The model under review builds one solid part; all positions refer to its coordinate system, in mm. Face numbers are marked on the shaded views. A direction names the side the tool comes from. Give positions to 0.01 mm unless a question says otherwise; leave off trailing zeros. Loops run counter-clockwise (first coordinate to the right, second up) from the corner with the lowest first, then second, coordinate; pieces in that order, holes last. Notation, with made-up numbers: M 51,4 L 84,4 A28 cw 84,31 Z; hole C 86.25,28.25 d1. An arc over 180 degrees is marked long. Return JSON: item names as keys, results as strings.
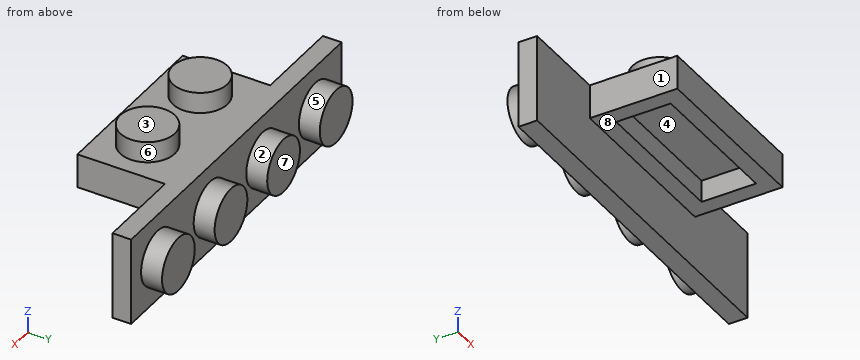
```python
from build123d import *

# Parameters (mm, degrees)
SKETCH1_W           = 15.9
SKETCH1_H           = 7.95
BOSS_EXTRUDE1_DEPTH = 3.1
SKETCH2_R           = 2.475
BOSS_EXTRUDE2_DEPTH = 1.9
SKETCH3_W           = 12.9
SKETCH3_H           = 4.95
CUT_EXTRUDE1_DEPTH  = 2
SKETCH4_W           = 31.8
SKETCH4_H           = 7.95
BOSS_EXTRUDE3_DEPTH = 1.7
SKETCH5_R           = 2.475
BOSS_EXTRUDE4_DEPTH = 1.9
LPATTERN1_COUNT     = 4
LPATTERN1_PITCH     = 7.95


with BuildPart() as part:
    # Sketch1 → Boss-Extrude1 (new body)
    with BuildSketch(Plane.XY):
        with Locations((7.95, -3.975)):
            Rectangle(SKETCH1_W, SKETCH1_H)
    extrude(amount=BOSS_EXTRUDE1_DEPTH)

    # Sketch2 → Boss-Extrude2 (add)
    with BuildSketch(Plane.XY.offset(3.1)):
        with Locations(Location((3.975, -3.975, 0), (0, 0, 180))):
            Circle(SKETCH2_R)
        with Locations(Location((11.925, -3.975, 0), (0, 0, 180))):
            Circle(SKETCH2_R)
    extrude(amount=BOSS_EXTRUDE2_DEPTH)

    # Sketch3 → Cut-Extrude1 (cut)
    with BuildSketch(Plane(origin=(0, 0, 0), x_dir=(-1, 0, 0), z_dir=(0, 0, -1))):
        with Locations((-7.95, -3.975)):
            Rectangle(SKETCH3_W, SKETCH3_H)
    extrude(amount=-CUT_EXTRUDE1_DEPTH, mode=Mode.SUBTRACT)

    # Sketch4 → Boss-Extrude3 (add)
    with BuildSketch(Plane(origin=(0, 0, 0), x_dir=(1, 0, 0), z_dir=(0, 1, 0))):
        with Locations((7.95, 0.875)):
            Rectangle(SKETCH4_W, SKETCH4_H)
    extrude(amount=BOSS_EXTRUDE3_DEPTH)

    # Sketch5 → Boss-Extrude4 (add)
    with BuildSketch(Plane(origin=(0, 1.7, 0), x_dir=(1, 0, 0), z_dir=(0, 1, 0))):
        with Locations(Location((-3.975, 0.875, 0), (0, 0, 90))):
            Circle(SKETCH5_R)
    boss_extrude4 = extrude(amount=BOSS_EXTRUDE4_DEPTH)

    # LPattern1: Boss-Extrude4 ×4
    with Locations(*[(i * LPATTERN1_PITCH, 0, 0) for i in range(1, LPATTERN1_COUNT)]):
        add(boss_extrude4)


solid = part.part
```
1) Tool access review of the marked faces 4, 5, 6, 7 and 8: name each direction out of +Z, -Z, +X, -X, +Y, -Y from which nothing blocks a thin tool from reaching the whole face with its end or side.
From the geometry:
{"face 4": "-Z", "face 5": "+Y", "face 6": "+Z", "face 7": "+Z, -Z, +X, -X, +Y", "face 8": "-Z, +X, -X, -Y"}
2) Insertion check: pin 1 (2 mm diameter, centred on y = -4, z = 1.5, fed in from -X); pin 2 (1.5 mm diameter, centred on x = 20, y = -1.5, fed in from +Z); pin 3 (1 mm diameter, centred on x = -2, z = -2, fed in from -Y); pin 4 (3 mm diameter, centred on x = -3, y = 1.5, fed in from +Z). Each pin has a flat end and moves straight along its axis. Give the tip position at first contact, or say it passes through.
From the geometry:
{"pin 1": "x = 0", "pin 2": "through", "pin 3": "y = 0", "pin 4": "z = 3.1"}
3) Consider section A-A on x = 8. Write out the cut boundary in (y, z), then the cut area to 3 significant figures.
From the geometry:
{"outline": "M -7.95,0 L -6.45,0 L -6.45,2 L -1.5,2 L -1.5,0 L 0,0 L 0,-4.85 L 1.7,-4.85 L 1.7,3.1 L -7.95,3.1 Z", "area": "28.3 mm²"}
4) Consider section B-B on z = -4.5. Write out the cut boundary in (x, y).
From the geometry:
{"outline": "M -7.95,0 L 23.85,0 L 23.85,1.7 L -7.95,1.7 Z"}
5) Consider section C-C on y = -2.25. Write out the cut boundary in (x, z).
From the geometry:
{"outline": "M 0,0 L 1.5,0 L 1.5,2 L 14.4,2 L 14.4,0 L 15.9,0 L 15.9,3.1 L 13.7,3.1 L 13.7,5 L 10.15,5 L 10.15,3.1 L 5.75,3.1 L 5.75,5 L 2.2,5 L 2.2,3.1 L 0,3.1 Z"}
6) The part is to be moulded in two halves that separate along X. For the marked faces 1, 2 and 3, say which applies: released by +X, released by -X, zero draft, split by the parting line, or undercut.
From the geometry:
{"face 1": "released by -X", "face 2": "undercut", "face 3": "zero draft"}
7) Wall thickness on L1, parallel to X at y = -5.5, z = 0.5; L2, parallel to X at y = -4, z = 4; L3, parallel to Z at x = 5, y = -5.75: over which ranges is each line inside the solid? List them lowest first. Write a range as from..to.
From the geometry:
{"L1": "0..1.5, 14.4..15.9", "L2": "1.5..6.45, 9.45..14.4", "L3": "2..5"}
8) Consider section D-D on z = 1. Write out the cut boundary in (x, y).
From the geometry:
{"outline": "M -7.95,0 L 0,0 L 0,-7.95 L 15.9,-7.95 L 15.9,0 L 23.85,0 L 23.85,1.7 L 21.49,1.7 L 21.49,3.6 L 18.26,3.6 L 18.26,1.7 L 13.54,1.7 L 13.54,3.6 L 10.31,3.6 L 10.31,1.7 L 5.59,1.7 L 5.59,3.6 L 2.36,3.6 L 2.36,1.7 L -2.36,1.7 L -2.36,3.6 L -5.59,3.6 L -5.59,1.7 L -7.95,1.7 Z; hole M 1.5,-6.45 L 14.4,-6.45 L 14.4,-1.5 L 1.5,-1.5 Z"}
